Read the model definition and answer for the solid it produces. Units are mm, in the model's axes. Round coordinates to 2 decimals unless told otherwise and drop trailing zeros. Order: outer loops, then holes, each group sorted by start corner. A loop starts at its lowest first (then second) coordinate and runs counter-clockwise, first axis right, second up. Notation, with made-up numbers: (85.5, -6) - (97.5, -6) arc R26 cw to (97.5, 14) - close; hole circle Ø11 at (-22.75, 39). An arc over 180 degrees is marked (long way). Answer as a JSON object with one key per item and string values. Group by question number.
Q1. Consider line 1 (Y direction, x = 290.75, z = 1); line 2 (X direction, y = -127, z = 2.85); line 3 (Y direction, x = 145.5, z = 1.1). Determine where each line is inside the solid, lowest interval first.
Q2. A cutting plane is placed at A-A on x = 192. Determine the outline of the cut face in (y, z).
Q3. A cutting plane is placed at B-B on x = 241. Determine the outline of the cut face in (y, z).
Q4. Given pin 1 Ø2 at (y, z) = (-258, 2.5) entering from -X; pin 2 Ø1.2 at (x, z) = (111.5, 2) entering from +Y; pin 3 Ø2 at (y, z) = (-251, 1) entering from +X, each flat-ended and moving along its own axis, determine where each tip first touches the part or whether it passes through.
Q5. A cutting plane is placed at C-C on z = 1.3. Count the separate pieces of the cut face and the enclosed holes in it, and give its area (3 significant figures).
Autodesk Inventor part; units mm, degrees
ref_plane "YZ Plane" through (0, 0, 0) normal (1, 0, 0) x (0, 1, 0)
ref_plane "XZ Plane" through (0, 0, 0) normal (0, 1, 0) x (-1, 0, 0)
ref_plane "XY Plane" through (0, 0, 0) normal (0, 0, 1) x (1, 0, 0)
sketch "Эскиз1" plane through (0, 0, 0) normal (0, 0, 1) x (1, 0, 0)
  line L0 (46, -47) -> (277, -47)
  line L1 (277, -47) -> (277, -333)
  line L2 (277, -333) -> (46, -333)
  line L3 (46, -333) -> (46, -47)
  line L4 (-2, 5) -> (334, 5)
  line L5 (338, 5) -> (338, -385)
  line L6 (334, -385) -> (-2, -385)
  line L7 (-6, -385) -> (-6, 5)
  line L8 (-6, 5) -> (338, 5)
  line L9 (338, 5) -> (338, -385)
  line L10 (338, -385) -> (-6, -385)
  line L11 (-6, -385) -> (-6, 5)
  dimension "d4" = 231
  dimension "d10" = 61
  dimension "d11" = 52
  dimension "d12" = 52
  dimension "d13" = 52
extrude "Выдавливание3" add sketch "Эскиз1" along normal blind 4
sketch "Эскиз3" plane through (0, 0, 4) normal (0, 0, 1) x (1, 0, 0)
  circle A0 centre (290.75, -97) radius 1.5
  circle A1 centre (290.75, -127) radius 1.5
  line L0 (46, -47) -> (277, -47)
  line L1 (277, -47) -> (277, -333)
  circle A2 centre (290.75, -253) radius 1.5
  circle A3 centre (290.75, -283) radius 1.5
  line L2 (277, -333) -> (46, -333)
  point P0 (0, 0)
  dimension "d19" = 3
  dimension "d20" = 3
  dimension "d21" = 30
  dimension "d22" = 50
  dimension "d23" = 13.75
  dimension "d24" = 13.75
  dimension "d25" = 3
  dimension "d26" = 3
  dimension "d27" = 30
  dimension "d28" = 13.75
  dimension "d29" = 13.75
  dimension "d30" = 50
extrude "Выдавливание4" cut sketch "Эскиз3" against normal blind 10
chamfer "Фаска1" distance 15 angle 45 4 edges at (277, -47, 2) (277, -333, 2) (46, -47, 2) (46, -333, 2)
sketch "Эскиз4" plane through (0, 0, 4) normal (0, 0, 1) x (1, 0, 0)
  ellipse E0 centre (40.9735, -191.8546) end of major axis (40.9735, -190.3546) minor radius 1.4997
  line L0 (40.9735, -191.8546) -> (10.6659, -191.8546) construction
  circle A0 centre (40.733, -191.8546) radius 1.5
  line L1 (46, -62) -> (46, -318)
  point P0 (0, 0)
  dimension "d36" = 3
  dimension "d37" = 5.267
extrude "Выдавливание5" cut sketch "Эскиз4" against normal blind 10 contours A0 E0 | E0 A0 picked at (41.2979, -191.9775) picked at (39.4227, -191.6148)
sketch "Эскиз5" plane through (0, 0, 4) normal (0, 0, 1) x (1, 0, 0)
  line L0 (-6, -73.3) -> (-2, -73.3)
  line L1 (-6, -150.7) -> (-2, -150.7)
  line L2 (-2, -73.3) -> (-2, -150.7)
  line L3 (-6, 5) -> (-6, -385)
  line L4 (-6, -229.3) -> (-2, -229.3)
  line L5 (-2, -229.3) -> (-2, -306.7)
  line L6 (-6, -306.7) -> (-2, -306.7)
  line L7 (63.3, -385) -> (63.3, -381)
  line L8 (133.2, -385) -> (63.3, -385)
  line L9 (133.2, -385) -> (133.2, -381)
  line L10 (63.3, -381) -> (133.2, -381)
  line L11 (63.3, -385) -> (63.3, -381)
  line L12 (268.7, -385) -> (198.8, -385)
  line L13 (268.7, -385) -> (268.7, -381)
  line L14 (198.8, -381) -> (268.7, -381)
  line L15 (198.8, -385) -> (198.8, -381)
  line L16 (63.3, 5) -> (133.2, 5)
  line L17 (63.3, 5) -> (63.3, 1)
  line L18 (133.2, 1) -> (63.3, 1)
  line L19 (133.2, 5) -> (133.2, 1)
  line L20 (198.8, 5) -> (268.7, 5)
  line L21 (198.8, 5) -> (198.8, 1)
  line L22 (268.7, 1) -> (198.8, 1)
  line L23 (268.7, 5) -> (268.7, 1)
  line L24 (338, -229.3) -> (334, -229.3)
  line L25 (334, -306.7) -> (334, -229.3)
  line L26 (338, -306.7) -> (334, -306.7)
  line L27 (338, -229.3) -> (338, -306.7)
  line L28 (338, -150.7) -> (334, -150.7)
  line L29 (338, -73.3) -> (338, -150.7)
  line L30 (334, -150.7) -> (334, -73.3)
  line L31 (338, -73.3) -> (334, -73.3)
  line L32 (63.1, 0.8) -> (63.1, 5.2)
  line L33 (63.1, 5.2) -> (133.4, 5.2)
  line L34 (133.4, 5.2) -> (133.4, 0.8)
  line L35 (133.4, 0.8) -> (63.1, 0.8)
  line L36 (198.6, 0.8) -> (198.6, 5.2)
  line L37 (198.6, 5.2) -> (268.9, 5.2)
  line L38 (268.9, 5.2) -> (268.9, 0.8)
  line L39 (268.9, 0.8) -> (198.6, 0.8)
  line L40 (333.8, -73.1) -> (333.8, -150.9)
  line L41 (333.8, -150.9) -> (338.2, -150.9)
  line L42 (338.2, -150.9) -> (338.2, -73.1)
  line L43 (338.2, -73.1) -> (333.8, -73.1)
  line L44 (333.8, -229.1) -> (338.2, -229.1)
  line L45 (338.2, -229.1) -> (338.2, -306.9)
  line L46 (338.2, -306.9) -> (333.8, -306.9)
  line L47 (333.8, -306.9) -> (333.8, -229.1)
  line L48 (268.9, -380.8) -> (268.9, -385.2)
  line L49 (268.9, -385.2) -> (198.6, -385.2)
  line L50 (198.6, -385.2) -> (198.6, -380.8)
  line L51 (198.6, -380.8) -> (268.9, -380.8)
  line L52 (133.2, -385) -> (63.3, -385)
  line L53 (133.2, -385) -> (133.2, -381)
  line L54 (63.3, -381) -> (133.2, -381)
  line L55 (63.3, -385) -> (63.3, -381)
  line L56 (63.3, -385) -> (63.3, -381)
  line L57 (63.3, -381) -> (133.2, -381)
  line L58 (-6, -306.9) -> (-1.8, -306.9)
  line L59 (-1.8, -306.9) -> (-1.8, -229.1)
  line L60 (-1.8, -229.1) -> (-6, -229.1)
  line L61 (-6, -150.9) -> (-1.8, -150.9)
  line L62 (-1.8, -150.9) -> (-1.8, -73.1)
  line L63 (-1.8, -73.1) -> (-6, -73.1)
  line L64 (-6, -73.1) -> (-6, -150.9)
  line L65 (-6, -229.1) -> (-6, -306.9)
  line L66 (63.3, -381) -> (133.2, -381)
  line L67 (133.2, -381) -> (133.2, -385)
  line L68 (133.2, -385) -> (63.3, -385)
  line L69 (63.3, -385) -> (63.3, -381)
  line L70 (63.3, -380.8) -> (133.2, -380.8)
  line L71 (63.1, -385) -> (63.1, -381)
  line L72 (133.4, -385) -> (133.4, -381)
  line L73 (133.4, -380.8) -> (63.1, -380.8)
  line L74 (63.1, -380.8) -> (63.1, -385.2)
  line L75 (63.1, -385.2) -> (133.4, -385.2)
  line L76 (133.4, -385.2) -> (133.4, -380.8)
  point P0 (0, 0)
  dimension "d40" = 4
  dimension "d41" = 69.9
  dimension "d42" = 69.9
  dimension "d43" = 0.2
  dimension "d44" = 0.2
  dimension "d45" = 0.2
  dimension "d46" = 0.2
  dimension "d47" = 0.2
  dimension "d48" = 0.2
  dimension "d49" = 0.2
  dimension "d50" = 0.2
  dimension "d51" = 0.2
  dimension "d52" = 0.2
extrude "Выдавливание6" cut sketch "Эскиз5" against normal blind 4.2 contours L3 L63 L62 L61 L1 L2 L0 | L60 L59 L58 L3 L6 L5 L4 | L0 L2 L1 L3 | L4 L5 L6 L3 | L7 L10 L9 L8 | L12 L15 L14 L13 | L16 L19 L18 L17 | L20 L23 L22 L21 | L27 L26 L25 L24 | L28 L30 L31 L29 | L32 L33 L34 L35 | L36 L37 L38 L39 | L43 L42 L41 L40 | L44 L45 L46 L47 | L48 L49 L50 L51 | L70 L73 L76 L72 L75 L74 L71
sketch "Эскиз6" plane through (0, 0, 4) normal (0, 0, 1) x (1, 0, 0)
  line L0 (302.85, -381) -> (302.85, -385)
  line L1 (299.85, -385) -> (299.85, -381)
  line L2 (167.5, -381) -> (167.5, -385)
  line L3 (164.5, -385) -> (164.5, -381)
  line L4 (32.15, -381) -> (32.15, -385)
  line L5 (29.15, -385) -> (29.15, -381)
  line L6 (301.35, -381) -> (301.35, -381)
  line L7 (166, -381) -> (166, -381)
  line L8 (30.65, -381) -> (30.65, -381)
  line L9 (63.1, -380.8) -> (133.4, -380.8)
  line L10 (302.85, -381) -> (299.85, -381)
  line L11 (299.85, -382.5) -> (299.85, -385)
  line L12 (299.85, -385) -> (302.85, -385)
  line L13 (302.85, -385) -> (302.85, -382.5)
  line L14 (167.5, -381) -> (164.5, -381)
  line L15 (164.5, -382.5) -> (164.5, -385)
  line L16 (164.5, -385) -> (167.5, -385)
  line L17 (167.5, -385) -> (167.5, -382.5)
  line L18 (32.15, -381) -> (29.15, -381)
  line L19 (29.15, -382.5) -> (29.15, -385)
  line L20 (29.15, -385) -> (32.15, -385)
  line L21 (32.15, -385) -> (32.15, -382.5)
  line L22 (334, -344.35) -> (338, -344.35)
  line L23 (338, -347.35) -> (334, -347.35)
  line L24 (334, -188.5) -> (338, -188.5)
  line L25 (338, -191.5) -> (334, -191.5)
  line L26 (334, -32.65) -> (338, -32.65)
  line L27 (338, -35.65) -> (334, -35.65)
  line L28 (302.85, 5) -> (302.85, 1)
  line L29 (299.85, 1) -> (299.85, 5)
  line L30 (167.5, 5) -> (167.5, 1)
  line L31 (164.5, 1) -> (164.5, 5)
  line L32 (32.15, 5) -> (32.15, 1)
  line L33 (29.15, 1) -> (29.15, 5)
  line L34 (-6, -32.65) -> (-2, -32.65)
  line L35 (-2, -35.65) -> (-6, -35.65)
  line L36 (-6, -188.5) -> (-2, -188.5)
  line L37 (-2, -191.5) -> (-6, -191.5)
  line L38 (-6, -344.35) -> (-2, -344.35)
  line L39 (-2, -347.35) -> (-6, -347.35)
  line L40 (338, -344.35) -> (335.5, -344.35)
  line L41 (334, -345.85) -> (334, -345.85)
  line L42 (335.5, -347.35) -> (338, -347.35)
  line L43 (338, -347.35) -> (338, -344.35)
  line L44 (338, -188.5) -> (335.5, -188.5)
  line L45 (334, -190) -> (334, -190)
  line L46 (335.5, -191.5) -> (338, -191.5)
  line L47 (338, -191.5) -> (338, -188.5)
  line L48 (338, -32.65) -> (335.5, -32.65)
  line L49 (334, -34.15) -> (334, -34.15)
  line L50 (335.5, -35.65) -> (338, -35.65)
  line L51 (338, -35.65) -> (338, -32.65)
  line L52 (302.85, 5) -> (299.85, 5)
  line L53 (299.85, 5) -> (299.85, 2.5)
  line L54 (301.35, 1) -> (301.35, 1)
  line L55 (302.85, 2.5) -> (302.85, 5)
  line L56 (167.5, 5) -> (164.5, 5)
  line L57 (164.5, 5) -> (164.5, 2.5)
  line L58 (166, 1) -> (166, 1)
  line L59 (167.5, 2.5) -> (167.5, 5)
  line L60 (32.15, 5) -> (29.15, 5)
  line L61 (29.15, 5) -> (29.15, 2.5)
  line L62 (30.65, 1) -> (30.65, 1)
  line L63 (32.15, 2.5) -> (32.15, 5)
  line L64 (-3.5, -32.65) -> (-6, -32.65)
  line L65 (-6, -32.65) -> (-6, -35.65)
  line L66 (-6, -35.65) -> (-3.5, -35.65)
  line L67 (-2, -34.15) -> (-2, -34.15)
  line L68 (-3.5, -188.5) -> (-6, -188.5)
  line L69 (-6, -188.5) -> (-6, -191.5)
  line L70 (-6, -191.5) -> (-3.5, -191.5)
  line L71 (-2, -190) -> (-2, -190)
  line L72 (-3.5, -344.35) -> (-6, -344.35)
  line L73 (-6, -344.35) -> (-6, -347.35)
  line L74 (-6, -347.35) -> (-3.5, -347.35)
  line L75 (-2, -345.85) -> (-2, -345.85)
  arc A0 (167.5, -382.5) -> (166, -381) centre (166, -382.5) ccw
  arc A1 (166, -381) -> (164.5, -382.5) centre (166, -382.5) ccw
  arc A2 (32.15, -382.5) -> (30.65, -381) centre (30.65, -382.5) ccw
  arc A3 (30.65, -381) -> (29.15, -382.5) centre (30.65, -382.5) ccw
  arc A4 (-2, -345.85) -> (-3.5, -344.35) centre (-3.5, -345.85) ccw
  arc A5 (-3.5, -347.35) -> (-2, -345.85) centre (-3.5, -345.85) ccw
  arc A6 (-2, -190) -> (-3.5, -188.5) centre (-3.5, -190) ccw
  arc A7 (-3.5, -191.5) -> (-2, -190) centre (-3.5, -190) ccw
  arc A8 (-2, -34.15) -> (-3.5, -32.65) centre (-3.5, -34.15) ccw
  arc A9 (-3.5, -35.65) -> (-2, -34.15) centre (-3.5, -34.15) ccw
  arc A10 (30.65, 1) -> (32.15, 2.5) centre (30.65, 2.5) ccw
  arc A11 (29.15, 2.5) -> (30.65, 1) centre (30.65, 2.5) ccw
  arc A12 (166, 1) -> (167.5, 2.5) centre (166, 2.5) ccw
  arc A13 (164.5, 2.5) -> (166, 1) centre (166, 2.5) ccw
  arc A14 (301.35, 1) -> (302.85, 2.5) centre (301.35, 2.5) ccw
  arc A15 (299.85, 2.5) -> (301.35, 1) centre (301.35, 2.5) ccw
  arc A16 (335.5, -32.65) -> (334, -34.15) centre (335.5, -34.15) ccw
  arc A17 (334, -34.15) -> (335.5, -35.65) centre (335.5, -34.15) ccw
  arc A18 (335.5, -188.5) -> (334, -190) centre (335.5, -190) ccw
  arc A19 (334, -190) -> (335.5, -191.5) centre (335.5, -190) ccw
  arc A20 (335.5, -344.35) -> (334, -345.85) centre (335.5, -345.85) ccw
  arc A21 (334, -345.85) -> (335.5, -347.35) centre (335.5, -345.85) ccw
  arc A22 (302.85, -382.5) -> (301.35, -381) centre (301.35, -382.5) ccw
  arc A23 (301.35, -381) -> (299.85, -382.5) centre (301.35, -382.5) ccw
  point P0 (0, 0)
  dimension "d55" = 1.5
  dimension "d56" = 1.5
extrude "Выдавливание7" cut sketch "Эскиз6" against normal blind 10 contours L0 L12 L1 A23 A22 | L2 L16 L3 A1 A0 | L4 L20 L5 A3 A2 | L22 L43 L23 A21 A20 | L24 L47 L25 A19 A18 | L26 L51 L27 A17 A16 | L28 A14 A15 L29 L52 | L30 A12 A13 L31 L56 | L32 A10 A11 L33 L60 | L34 A8 A9 L35 L65 | L36 A6 A7 L37 L69 | L38 A4 A5 L39 L73
properties part number "крышка"
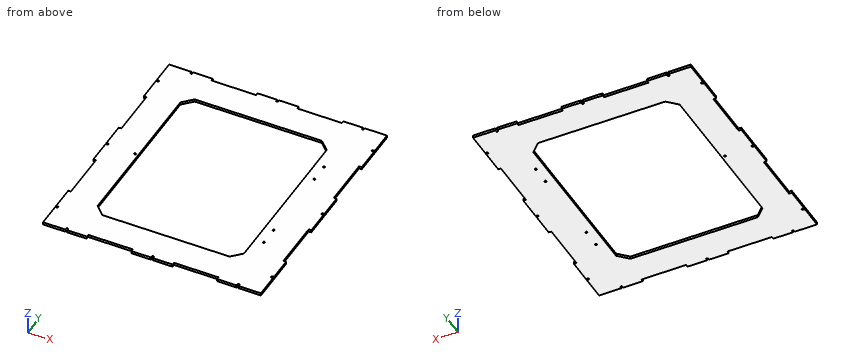
Result set:
{
 "1": {"line 1": "y = -385 to -284.5, -281.5 to -254.5, -251.5 to -128.5, -125.5 to -98.5, -95.5 to 5", "line 2": "x = -1.8 to 46, 277 to 289.25, 292.25 to 333.8", "line 3": "y = -385 to -333, -47 to 5"},
 "2": {"outline": "(-385, 0) - (-333, 0) - (-333, 4) - (-385, 4) - close; (-47, 0) - (5, 0) - (5, 4) - (-47, 4) - close"},
 "3": {"outline": "(-380.8, 0) - (-333, 0) - (-333, 4) - (-380.8, 4) - close; (-47, 0) - (0.8, 0) - (0.8, 4) - (-47, 4) - close"},
 "4": {"pin 1": "stops at x = -1.8", "pin 2": "stops at y = 0.8", "pin 3": "stops at x = 333.8"},
 "5": {"separate pieces": "1", "enclosed holes": "6", "area": "65,900 mm²"}
}
